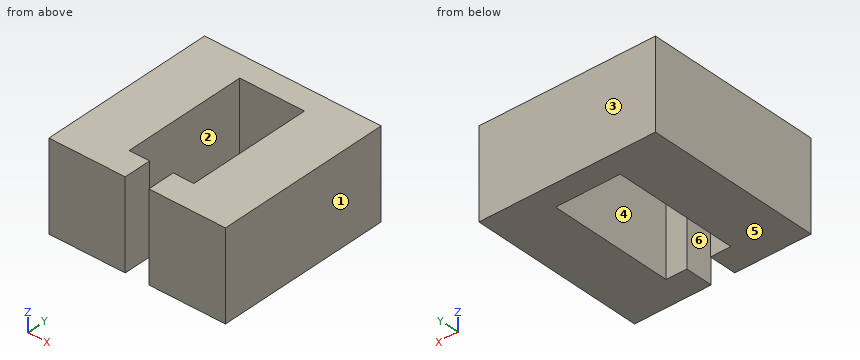
from build123d import *

# Parameters (mm, degrees)
SKETCH1_W           = 60
SKETCH1_H           = 60
BOSS_EXTRUDE1_DEPTH = 30
SKETCH2_W           = 22
SKETCH2_H           = 42.6
CUT_EXTRUDE1_DEPTH  = 59.89947825
SKETCH4_W           = 8.015676437
SKETCH4_H           = 9.4
CUT_EXTRUDE3_DEPTH  = 59.89947825


with BuildPart() as part:
    # Sketch1 → Boss-Extrude1 (new body)
    with BuildSketch(Plane(origin=(0, 0, 7.302957559), x_dir=(-1, 0, 0), z_dir=(0, 0, -1))):
        with Locations((-2.674729751, 8.74932998)):
            Rectangle(SKETCH1_W, SKETCH1_H)
    extrude(amount=BOSS_EXTRUDE1_DEPTH)

    # Sketch2 → Cut-Extrude1 (cut, through all)
    with BuildSketch(Plane(origin=(0, 0, -22.697042441), x_dir=(-1, 0, 0), z_dir=(0, 0, -1))):
        with Locations((-2.674729751, 9.44932998)):
            Rectangle(SKETCH2_W, SKETCH2_H)
    extrude(amount=-CUT_EXTRUDE1_DEPTH, mode=Mode.SUBTRACT)

    # Sketch4 → Cut-Extrude3 (cut, through all)
    with BuildSketch(Plane(origin=(0, 0, -22.697042441), x_dir=(-1, 0, 0), z_dir=(0, 0, -1))):
        with Locations((-2.616126324, -16.55067002)):
            Rectangle(SKETCH4_W, SKETCH4_H)
    extrude(amount=-CUT_EXTRUDE3_DEPTH, mode=Mode.SUBTRACT)


solid = part.part
Check sheet for the modelled part. Datum: model origin and axes. Units: mm. Face numbers are marked on the shaded views. A direction names the side the tool comes from. Give positions to 0.01 mm unless a question says otherwise; leave off trailing zeros. Write each loop counter-clockwise with the first axis right and the second up, starting at its lowest first coordinate (ties: lowest second). Pieces come first, ordered by that corner, then holes. Notation, with made-up numbers: (74.25, 2.25) -> (94.25, 2.25) arc R27 ccw to (94.25, 23.25) -> close; hole circle Ø4 at (13, 70). An arc over 180 degrees is marked (long way). One line per item, written item: value. Start each with the question number.
Item 1: Draft check along X on the marked faces 1, 2 and 3. Enter one of: +X half, -X half, draft (parallel to the pull), parting line (faces both ways), or undercut.
Item 2: Gauge pin test, flat end, axial feed: pin 1 (4 mm diameter, centred on x = 5, z = -1.5, fed in from -Y). Record the tip position at first contact, or that the pin passes through.
Item 3: Material ranges on probe 1 along X at (y, z) = (3, 5.5); probe 2 along X at (y, z) = (-17.5, -12.5); probe 3 along Y at (x, z) = (-4.5, -19.25), recorded low to high. Write a range as from..to.
Item 4: Section check D-D on x = 3. Record the cut outline in (y, z), then the cut area to 3 significant figures.
Item 5: Section check C-C on z = -17.5. Record the cut outline in (x, y), then the cut area to 3 significant figures.
Item 6: Section check B-B on x = -3.5. Record the cut outline in (y, z), then the cut area to 3 significant figures.
Item 7: Section check A-A on y = 23. Record the cut outline in (x, z), then the cut area to 3 significant figures.
Item 8: Tool access check on the marked faces 4, 5 and 6. Record the directions out of +Z, -Z, +X, -X, +Y, -Y that give a thin tool (end or side, any length) a straight path to the whole face; none if there is none.
Results list:
1. face 1: +X half
1. face 2: undercut
1. face 3: draft
2. pin 1: y = -21.25
3. probe 1: -27.33..-8.33, 13.67..32.67
3. probe 2: -27.33..-1.39, 6.62..32.67
3. probe 3: -21.25..-11.85, 30.75..38.75
4. outline: (30.75, -22.7) -> (38.75, -22.7) -> (38.75, 7.3) -> (30.75, 7.3) -> close
4. area: 240 mm²
5. outline: (-27.33, -21.25) -> (-1.39, -21.25) -> (-1.39, -11.85) -> (-8.33, -11.85) -> (-8.33, 30.75) -> (13.67, 30.75) -> (13.67, -11.85) -> (6.62, -11.85) -> (6.62, -21.25) -> (32.67, -21.25) -> (32.67, 38.75) -> (-27.33, 38.75) -> close
5. area: 2,590 mm²
6. outline: (-21.25, -22.7) -> (-11.85, -22.7) -> (-11.85, 7.3) -> (-21.25, 7.3) -> close; (30.75, -22.7) -> (38.75, -22.7) -> (38.75, 7.3) -> (30.75, 7.3) -> close
6. area: 522 mm²
7. outline: (-27.33, -22.7) -> (-8.33, -22.7) -> (-8.33, 7.3) -> (-27.33, 7.3) -> close; (13.67, -22.7) -> (32.67, -22.7) -> (32.67, 7.3) -> (13.67, 7.3) -> close
7. area: 1,140 mm²
8. face 4: +Z, -Z
8. face 5: -Z, +X, -X, +Y, -Y
8. face 6: +Z, -Z, -Y
